Part model, mm, in its own coordinate system. Round coordinates to 2 decimals unless told otherwise and drop trailing zeros. Order: outer loops, then holes, each group sorted by start corner. A loop starts at its lowest first (then second) coordinate and runs counter-clockwise, first axis right, second up. Notation, with made-up numbers: M 71.25,11.25 L 128.25,11.25 A15 ccw 128.25,29.25 Z; hole C 74.25,-9 d9. An arc over 180 degrees is marked long. Write each question's results on one line, items separated by ' | '. Start each with the question number.
1. Band-saw the part on A-A, the plane y = -1.65. List the corners of the cut face in (x, z).
2. Drop flat-ended pins along their axis: pin 1 Ø1.4 at (y, z) = (-1.5, 9) entering from +X; pin 2 Ø0.5 at (x, y) = (-2, -2) entering from +Z; pin 3 Ø1.4 at (y, z) = (-1.5, 11.5) entering from -X. Give the stop position or say it passes through.
3. Probe L1, parallel to Z at x = 41.5, y = -0.7; L2, parallel to X at y = -2.55, z = 8; L3, parallel to X at y = -1.5, z = 14. List the from-to ranges inside material, lowest first. Write a range as [from, to].
4. Band-saw the part on C-C, the plane z = 7.5. List the corners of the cut face in (x, y).
5. Band-saw the part on B-B, the plane x = -4.5. List the corners of the cut face in (y, z), then the cut area to 3 significant figures.
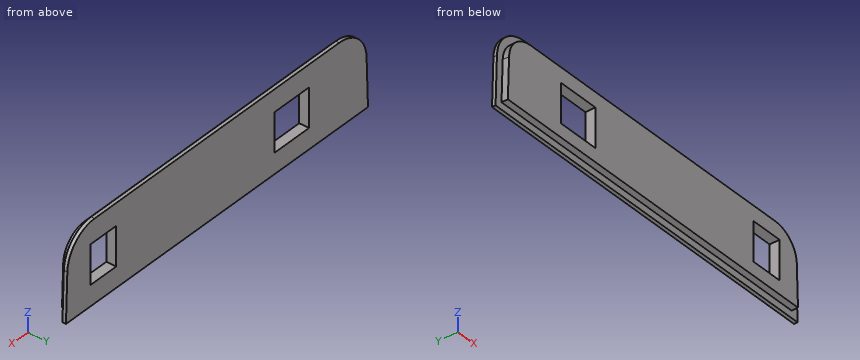
```python
from build123d import *

# Parameters (mm, degrees)
F1_DEPTH = 1
F3_DEPTH = 1.8
F4_W     = 9
F4_H     = 11
F4_W_2   = 12
F5_DEPTH = 2.801


with BuildPart() as f1:
    # F0 (on Front) → F1 (new body)
    with BuildSketch(Plane.XZ):
        with BuildLine():
            Line((-48.502349, 13.831545), (-48.985357, 0))
            Line((-48.985357, 0), (56.014643, 0))
            Line((56.014643, 0), (55.531635, 13.831545))
            ThreePointArc((55.531635, 13.831545), (52.636676, 20.333728), (46.037422, 23))
            Line((46.037422, 23), (-39.008136, 23))
            ThreePointArc((-39.008136, 23), (-45.607391, 20.333728), (-48.502349, 13.831545))
        make_face()
    extrude(amount=F1_DEPTH)

    # F2 (on face) → F3 (join)
    with BuildSketch(Plane.XZ.offset(1)):
        with BuildLine():
            Line((46.037422, 21), (-39.008136, 21))
            ThreePointArc((-39.008136, 21), (-44.218074, 18.895049), (-46.503567, 13.761746))
            Line((-46.503567, 13.761746), (-46.914297, 2))
            Line((-46.914297, 2), (53.943582, 2))
            Line((53.943582, 2), (53.532853, 13.761746))
            ThreePointArc((53.532853, 13.761746), (51.24736, 18.895049), (46.037422, 21))
        make_face()
    extrude(amount=F3_DEPTH)

    # F4 (on face) → F5 (cut, through all)
    with BuildSketch(Plane(origin=(0, 0, 0), x_dir=(-1, 0, 0), z_dir=(0, 1, 0))):
        with Locations((-43.031635, 11.3)):
            Rectangle(F4_W, F4_H)
        with Locations((22.502349, 11.3)):
            Rectangle(F4_W_2, F4_H)
    extrude(amount=-F5_DEPTH, mode=Mode.SUBTRACT)


solid = f1.part
```
Solution:
1) outline: M -46.91,2 L 53.94,2 L 53.53,13.76 A7.5 ccw 46.04,21 L -39.01,21 A7.5 ccw -46.5,13.76 Z; hole M -28.5,5.8 L -16.5,5.8 L -16.5,16.8 L -28.5,16.8 Z; hole M 38.53,5.8 L 47.53,5.8 L 47.53,16.8 L 38.53,16.8 Z
2) pin 1: x = 55.72 | pin 2: z = 21 | pin 3: x = -48.6
3) L1: [0, 5.8], [16.8, 23] | L2: [-46.7, -28.5], [-16.5, 38.53], [47.53, 53.73] | L3: [-46.49, -28.5], [-16.5, 38.53], [47.53, 53.52]
4) outline: M -48.72,-1 L -46.72,-1 L -46.72,-2.8 L -28.5,-2.8 L -28.5,0 L -48.72,0 Z; M -16.5,-2.8 L 38.53,-2.8 L 38.53,0 L -16.5,0 Z; M 47.53,-2.8 L 53.75,-2.8 L 53.75,-1 L 55.75,-1 L 55.75,0 L 47.53,0 Z
5) outline: M -2.8,2 L -1,2 L -1,0 L 0,0 L 0,23 L -1,23 L -1,21 L -2.8,21 Z | area: 57.2 mm^2
